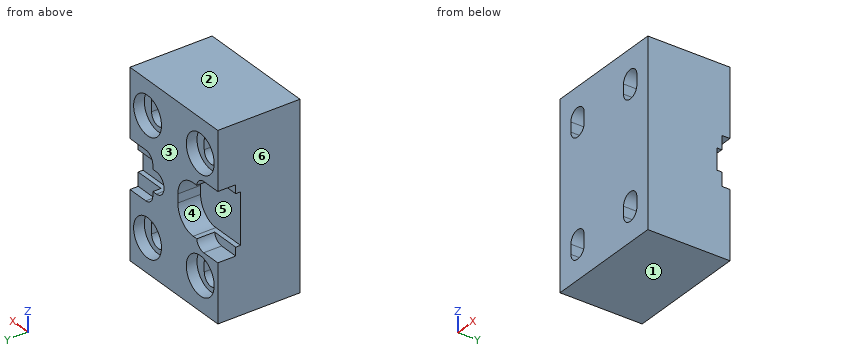
from build123d import *

# Parameters (mm, degrees)
SKETCH1_W                                           = 25
SKETCH1_H                                           = 38
BOSS_EXTRUDE1_DEPTH                                 = 17
CUT_EXTRUDE3_DEPTH                                  = 3.7
CUT_EXTRUDE4_DEPTH                                  = 1.7
CBORE_FOR_6_BINDING_HEAD_MACHINE_SCREW1_D           = 3.7973
CBORE_FOR_6_BINDING_HEAD_MACHINE_SCREW1_CBORE_D     = 7.9375
CBORE_FOR_6_BINDING_HEAD_MACHINE_SCREW1_CBORE_DEPTH = 2.2098
SKETCH12_W                                          = 1
SKETCH12_H                                          = 4.37
SKETCH12_W_2                                        = 6.5
CUT_EXTRUDE5_DEPTH                                  = 2.7
CUT_EXTRUDE6_DEPTH                                  = 4.7
CUT_EXTRUDE7_DEPTH                                  = 21682.908892909


with BuildPart() as part:
    # Sketch1 → Boss-Extrude1 (new body)
    with BuildSketch(Plane(origin=(0, 0, 0), x_dir=(1, 0, 0), z_dir=(0, 1, 0))):
        with Locations((-18481.446731235, 11298.191283293)):
            Rectangle(SKETCH1_W, SKETCH1_H)
    extrude(amount=BOSS_EXTRUDE1_DEPTH)

    # Sketch2 → Cut-Extrude3 (cut)
    with BuildSketch(Plane(origin=(0, 17, 0), x_dir=(1, 0, 0), z_dir=(0, 1, 0))):
        with BuildLine():
            Line((-18493.946731235, 11291.191283293), (-18489.946731235, 11291.191283293))
            ThreePointArc((-18489.946731235, 11291.191283293), (-18488.532517672, 11291.777069731), (-18487.946731235, 11293.191283293))
            Line((-18487.946731235, 11293.191283293), (-18487.946731235, 11303.191283293))
            ThreePointArc((-18487.946731235, 11303.191283293), (-18488.532517672, 11304.605496855), (-18489.946731235, 11305.191283293))
            Line((-18489.946731235, 11305.191283293), (-18493.946731235, 11305.191283293))
            Line((-18493.946731235, 11305.191283293), (-18493.946731235, 11291.191283293))
        make_face()
    extrude(amount=-CUT_EXTRUDE3_DEPTH, mode=Mode.SUBTRACT)

    # Sketch2<6> → Cut-Extrude4 (cut)
    with BuildSketch(Plane(origin=(0, 17, 0), x_dir=(1, 0, 0), z_dir=(0, 1, 0))):
        with BuildLine():
            Line((-18475.446731235, 11301.191283293), (-18475.446731235, 11295.191283293))
            ThreePointArc((-18475.446731235, 11295.191283293), (-18474.860944797, 11293.777069731), (-18473.446731235, 11293.191283293))
            Line((-18473.446731235, 11293.191283293), (-18468.946731235, 11293.191283293))
            Line((-18468.946731235, 11293.191283293), (-18468.946731235, 11303.191283293))
            Line((-18468.946731235, 11303.191283293), (-18473.446731235, 11303.191283293))
            ThreePointArc((-18473.446731235, 11303.191283293), (-18474.860944797, 11302.605496855), (-18475.446731235, 11301.191283293))
        make_face()
    extrude(amount=-CUT_EXTRUDE4_DEPTH, mode=Mode.SUBTRACT)

    # CBORE for #6 Binding Head Machine Screw1 (through all)
    with Locations(Plane(origin=(0, 17, 0), x_dir=(1, 0, 0), z_dir=(0, 1, 0))):
        with Locations((-18488.946731235, 11310.191283293), (-18473.946731235, 11310.191283293), (-18473.946731235, 11286.191283293), (-18488.946731235, 11286.191283293)):
            CounterBoreHole(CBORE_FOR_6_BINDING_HEAD_MACHINE_SCREW1_D / 2, CBORE_FOR_6_BINDING_HEAD_MACHINE_SCREW1_CBORE_D / 2, CBORE_FOR_6_BINDING_HEAD_MACHINE_SCREW1_CBORE_DEPTH)

    # Sketch12 → Cut-Extrude5 (cut)
    with BuildSketch(Plane(origin=(0, 17, 0), x_dir=(1, 0, 0), z_dir=(0, 1, 0))):
        with BuildLine():
            Line((-18476.446731235, 11300.376283293), (-18476.446731235, 11296.006283293))
            ThreePointArc((-18476.446731235, 11296.006283293), (-18478.631731235, 11298.191283293), (-18476.446731235, 11300.376283293))
        make_face()
        with Locations((-18475.946731235, 11298.191283293)):
            Rectangle(SKETCH12_W, SKETCH12_H)
        with Locations((-18472.196731235, 11298.191283293)):
            Rectangle(SKETCH12_W_2, SKETCH12_H)
    extrude(amount=-CUT_EXTRUDE5_DEPTH, mode=Mode.SUBTRACT)

    # Sketch13 → Cut-Extrude6 (cut)
    with BuildSketch(Plane(origin=(0, 17, 0), x_dir=(1, 0, 0), z_dir=(0, 1, 0))):
        with BuildLine():
            ThreePointArc((-18486.936731235, 11303.441283293), (-18483.853745669, 11302.164268859), (-18482.576731235, 11299.081283293))
            Line((-18482.576731235, 11299.081283293), (-18482.576731235, 11297.301283293))
            ThreePointArc((-18482.576731235, 11297.301283293), (-18483.853745669, 11294.218297727), (-18486.936731235, 11292.941283293))
            Line((-18486.936731235, 11292.941283293), (-18486.946731235, 11292.941283293))
            Line((-18486.946731235, 11292.941283293), (-18486.946731235, 11303.441283293))
            Line((-18486.946731235, 11303.441283293), (-18486.936731235, 11303.441283293))
        make_face()
        with BuildLine():
            ThreePointArc((-18487.946731235, 11303.191283293), (-18487.950656716, 11303.316529118), (-18487.962417752, 11303.441283293))
            Line((-18487.962417752, 11303.441283293), (-18493.946731235, 11303.441283293))
            Line((-18493.946731235, 11303.441283293), (-18493.946731235, 11292.941283293))
            Line((-18493.946731235, 11292.941283293), (-18487.962417752, 11292.941283293))
            ThreePointArc((-18487.962417752, 11292.941283293), (-18487.950656716, 11293.066037468), (-18487.946731235, 11293.191283293))
            Line((-18487.946731235, 11293.191283293), (-18487.946731235, 11303.191283293))
        make_face()
        with BuildLine():
            Line((-18486.946731235, 11292.941283293), (-18486.946731235, 11303.441283293))
            Line((-18486.946731235, 11303.441283293), (-18487.962417752, 11303.441283293))
            ThreePointArc((-18487.962417752, 11303.441283293), (-18487.950656716, 11303.316529118), (-18487.946731235, 11303.191283293))
            Line((-18487.946731235, 11303.191283293), (-18487.946731235, 11293.191283293))
            ThreePointArc((-18487.946731235, 11293.191283293), (-18487.950656716, 11293.066037468), (-18487.962417752, 11292.941283293))
            Line((-18487.962417752, 11292.941283293), (-18486.946731235, 11292.941283293))
        make_face()
    extrude(amount=-CUT_EXTRUDE6_DEPTH, mode=Mode.SUBTRACT)

    # Sketch14 → Cut-Extrude7 (cut, through all)
    with BuildSketch(Plane(origin=(0, 17, 0), x_dir=(1, 0, 0), z_dir=(0, 1, 0))):
        with BuildLine():
            Line((-18487.046731235, 11309.191283293), (-18487.046731235, 11311.191283293))
            ThreePointArc((-18487.046731235, 11311.191283293), (-18488.946731235, 11313.091283293), (-18490.846731235, 11311.191283293))
            Line((-18490.846731235, 11311.191283293), (-18490.846731235, 11309.191283293))
            ThreePointArc((-18490.846731235, 11309.191283293), (-18488.946731235, 11307.291283293), (-18487.046731235, 11309.191283293))
        make_face()
        with BuildLine():
            ThreePointArc((-18475.846731235, 11311.191283293), (-18473.946731235, 11313.091283293), (-18472.046731235, 11311.191283293))
            Line((-18472.046731235, 11311.191283293), (-18472.046731235, 11309.191283293))
            ThreePointArc((-18472.046731235, 11309.191283293), (-18473.946731235, 11307.291283293), (-18475.846731235, 11309.191283293))
            Line((-18475.846731235, 11309.191283293), (-18475.846731235, 11311.191283293))
        make_face()
        with BuildLine():
            ThreePointArc((-18487.046731235, 11285.191283293), (-18488.946731235, 11283.291283293), (-18490.846731235, 11285.191283293))
            Line((-18490.846731235, 11285.191283293), (-18490.846731235, 11287.191283293))
            ThreePointArc((-18490.846731235, 11287.191283293), (-18488.946731235, 11289.091283293), (-18487.046731235, 11287.191283293))
            Line((-18487.046731235, 11287.191283293), (-18487.046731235, 11285.191283293))
        make_face()
        with BuildLine():
            Line((-18475.846731235, 11287.191283293), (-18475.846731235, 11285.191283293))
            ThreePointArc((-18475.846731235, 11285.191283293), (-18473.946731235, 11283.291283293), (-18472.046731235, 11285.191283293))
            Line((-18472.046731235, 11285.191283293), (-18472.046731235, 11287.191283293))
            ThreePointArc((-18472.046731235, 11287.191283293), (-18473.946731235, 11289.091283293), (-18475.846731235, 11287.191283293))
        make_face()
    extrude(amount=-CUT_EXTRUDE7_DEPTH, mode=Mode.SUBTRACT)


solid = part.part
Work out the finished part from the listing and answer in its coordinate system (mm). Face numbers are marked on the shaded views. A direction names the side the tool comes from. Give positions to 0.01 mm unless a question says otherwise; leave off trailing zeros. Order: outer loops, then holes, each group sorted by start corner. A loop starts at its lowest first (then second) coordinate and runs counter-clockwise, first axis right, second up. Notation, with made-up numbers: (65, -33.5) -> (103, -33.5) arc R23 cw to (103, -6.5) -> close; hole circle Ø2 at (-14.5, 40). An arc over 180 degrees is marked (long way). One line per item, written item: value.
Item 1: A tool of negligible diameter and unlimited length cuts with its end or side. For the marked faces 5 and 6, from which of +Z, -Z, +X, -X, +Y, -Y can it reach the whole face along a straight path? Write none if from no direction.
Answer sheet:
face 5: -X, +Y
face 6: +Z, -Z, -X, +Y, -Y
Item 2: Straight lines are drawn through the part: probe 1 along X at (y, z) = (3, -11286); probe 2 along X at (y, z) = (10.5, -11308.5); probe 3 along Z at (x, y) = (-18487.5, 5.5). For each, find the intervals that lie inside material, in ascending order.
Answer sheet:
probe 1: -18493.95 to -18490.85, -18487.05 to -18475.85, -18472.05 to -18468.95
probe 2: -18493.95 to -18490.72, -18487.18 to -18475.72, -18472.18 to -18468.95
probe 3: -11317.19 to -11312.42, -11307.96 to -11288.42, -11283.96 to -11279.19
Item 3: Find section C-C, the plane z = -11302.5. Give the vertices of the cut face in (x, y).
Answer sheet:
outline: (-18493.95, 0) -> (-18468.95, 0) -> (-18468.95, 15.3) -> (-18474.96, 15.3) -> (-18474.96, 17) -> (-18484.23, 17) -> (-18484.23, 12.3) -> (-18493.95, 12.3) -> close
Item 4: Flat-ended cylindrical pins translate along their axes: P1, Ø4, axis at x = -18474, z = -11310.5, coming from the +Y side; P2, Ø3, axis at x = -18473, z = -11302.5, coming from the +Y side; P3, Ø0.7, axis at y = 16, z = -11295.5, coming from the +X side; P4, Ø1.4, axis at x = -18471, z = -11294.5, coming from the +Y side. Find the tip coordinate at first contact, or state that the pin passes through.
Answer sheet:
P1: y = 14.79
P2: y = 17
P3: x = -18475.45
P4: y = 15.3
Item 5: Find section B-B, the plane z = -11284. Give the vertices of the cut face in (x, y).
Answer sheet:
outline: (-18493.95, 0) -> (-18490.43, 0) -> (-18490.43, 14.79) -> (-18492.26, 14.79) -> (-18492.26, 17) -> (-18493.95, 17) -> close; (-18487.47, 0) -> (-18475.43, 0) -> (-18475.43, 14.79) -> (-18477.26, 14.79) -> (-18477.26, 17) -> (-18485.64, 17) -> (-18485.64, 14.79) -> (-18487.47, 14.79) -> close; (-18472.47, 0) -> (-18468.95, 0) -> (-18468.95, 17) -> (-18470.64, 17) -> (-18470.64, 14.79) -> (-18472.47, 14.79) -> close
Item 6: Determine the mould class of the marked faces 1, 2, 3 and 4 for opening direction Z: released by +Z, released by -Z, zero draft, split by the parting line, or undercut.
Answer sheet:
face 1: released by -Z
face 2: released by +Z
face 3: zero draft
face 4: undercut
Item 7: Find section D-D, the plane y = 13.75. State how many separate pieces and enclosed holes the cut face has, plus the area to 3 significant figures.
Answer sheet:
separate pieces: 1
enclosed holes: 4
area: 744 mm²
Item 8: Find section A-A, the plane y = 4.25. Give the vertices of the cut face in (x, z), plus the area to 3 significant figures.
Answer sheet:
outline: (-18493.95, -11317.19) -> (-18468.95, -11317.19) -> (-18468.95, -11279.19) -> (-18493.95, -11279.19) -> close; hole (-18490.85, -11311.19) arc R1.9 ccw to (-18487.05, -11311.19) -> (-18487.05, -11309.19) arc R1.9 ccw to (-18490.85, -11309.19) -> close; hole (-18490.85, -11287.19) arc R1.9 ccw to (-18487.05, -11287.19) -> (-18487.05, -11285.19) arc R1.9 ccw to (-18490.85, -11285.19) -> close; hole (-18475.85, -11311.19) arc R1.9 ccw to (-18472.05, -11311.19) -> (-18472.05, -11309.19) arc R1.9 ccw to (-18475.85, -11309.19) -> close; hole (-18475.85, -11287.19) arc R1.9 ccw to (-18472.05, -11287.19) -> (-18472.05, -11285.19) arc R1.9 ccw to (-18475.85, -11285.19) -> close
area: 874 mm²
